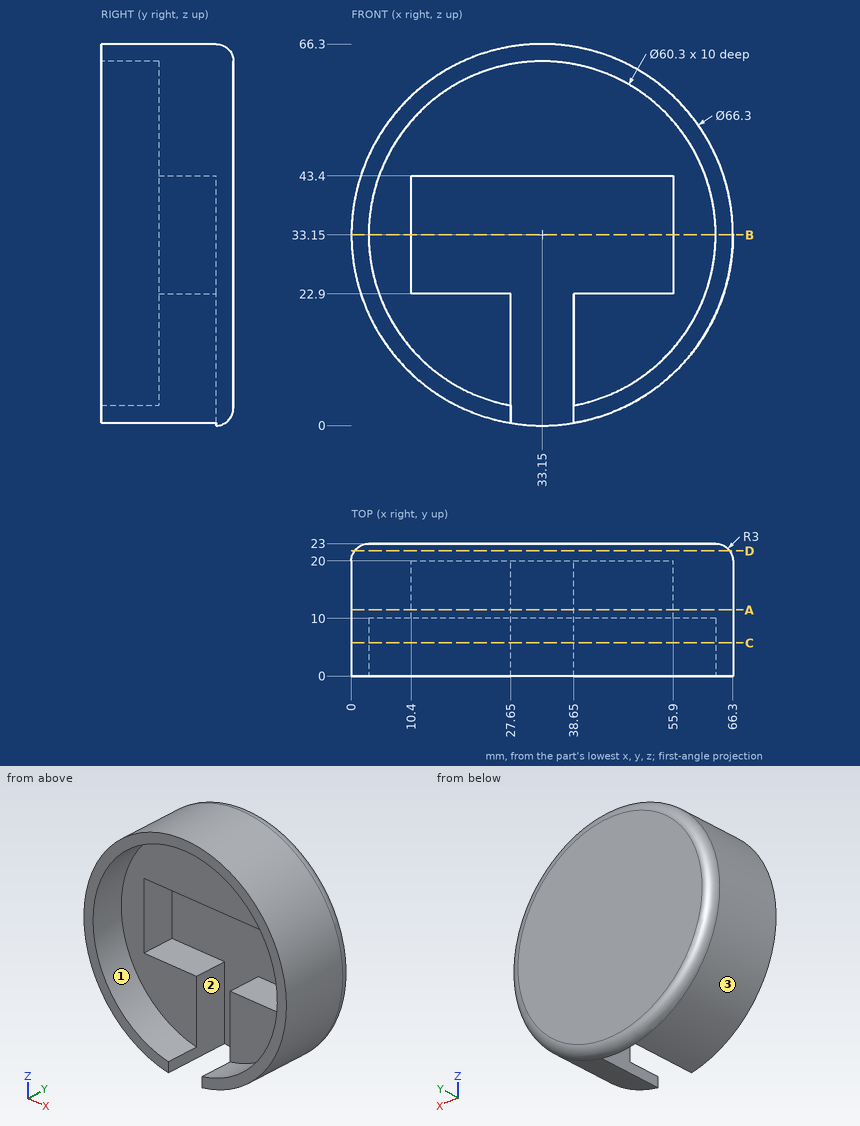
For this review, use the dimensioned drawing (mm, ordinates from the lowest corner) and the shaded views. A direction names the side the tool comes from. Coordinates: 2 decimals unless noted, no trailing zeros. Write each loop counter-clockwise with the first axis right and the second up, starting at its lowest first coordinate (ties: lowest second). Pieces come first, ordered by that corner, then holes. Notation, with made-up numbers: (63, -33.5) -> (95, -33.5) arc R29 cw to (95, -4.5) -> close; hole circle Ø3 at (15, -3). An arc over 180 degrees is marked (long way). Write each question's results on one line, items separated by ' | '. Start each with the question number.
(1) For line 1 along X through (y, z) = (3.75, 33.15); line 2 along Z through (x, y) = (33.15, 7.5); line 3 along X through (y, z) = (18.75, 40.5), list the stretches that pass through material, from the lowest coordinate up. Write a range as from..to.
(2) Clearance check with flat-ended pins moving along their axes: P1, Ø8, axis at y = 2.5, z = 34.5, coming from the -X side; P2, Ø8, axis at y = 4.5, z = 55.5, coming from the -X side; P3, Ø4, axis at y = 14, z = 24, coming from the +X side; P4, Ø6, axis at x = 20, z = 29, coming from the -Y side. State where each tip first meets the part, or that it passes through.
(3) Take a section at A-A on y = 11.5. Write out the cut boundary in (x, z).
(4) Take a section at C-C on y = 5.75. Write out the cut boundary in (x, z).
(5) Tool access review of the marked faces 1, 2 and 3: name each direction out of +Z, -Z, +X, -X, +Y, -Y from which nothing blocks a thin tool from reaching the whole face with its end or side.
(6) Take a section at D-D on y = 21.75. Write out the cut boundary in (x, z).
(7) Take a section at B-B on z = 33.15. Write out the cut boundary in (x, y).
Results found:
1) line 1: x = 0..3, 63.3..66.3 | line 2: z = 63.3..66.3 | line 3: x = 0.83..10.4, 55.9..65.47
2) P1: stops at x = 0 | P2: stops at x = 5.54 | P3: stops at x = 65.52 | P4: stops at y = 20
3) outline: (10.4, 22.9) -> (10.4, 43.4) -> (55.9, 43.4) -> (55.9, 22.9) -> (38.65, 22.9) -> (38.65, 0.46) arc R33.15 ccw (long way) to (27.65, 0.46) -> (27.65, 22.9) -> close
4) outline: (27.65, 0.46) -> (27.65, 3.51) arc R30.15 cw (long way) to (38.65, 3.51) -> (38.65, 0.46) arc R33.15 ccw (long way) to start
5) face 1: -Y | face 2: -Z, -Y | face 3: +Y, -Y
6) outline: circle Ø65.17 at (33.15, 33.15)
7) outline: (0, 0) -> (3, 0) -> (3, 10) -> (10.4, 10) -> (10.4, 20) -> (55.9, 20) -> (55.9, 10) -> (63.3, 10) -> (63.3, 0) -> (66.3, 0) -> (66.3, 20) arc R3 ccw to (63.3, 23) -> (3, 23) arc R3 ccw to (0, 20) -> close
